from build123d import *

# Parameters (mm, degrees)
SKETCH1_W                 = 37.50000004
SKETCH1_H                 = 31.999999963
BOSS_EXTRUDE1_DEPTH       = 3
SKETCH2_W                 = 6
SKETCH2_H                 = 61.71460232
BOSS_EXTRUDE2_DEPTH       = 25.662738028
SKETCH3_W                 = 63.162738068
SKETCH3_H                 = 6
BOSS_EXTRUDE3_DEPTH       = 5.000000037
SKETCH4_W                 = 63.162738068
SKETCH4_H                 = 6
BOSS_EXTRUDE4_DEPTH       = 8
SKETCH5_W                 = 6
SKETCH5_H                 = 74.714602357
BOSS_EXTRUDE5_DEPTH       = 55.76390052
CUT_EXTRUDE1_DEPTH        = 2.499999998
SKETCH7_W                 = 6
SKETCH7_H                 = 32.514602357
CUT_EXTRUDE2_DEPTH        = 18.3
SKETCH8_W                 = 6
SKETCH8_H                 = 29.714602357
CUT_EXTRUDE3_DEPTH        = 2.5
SKETCH9_W                 = 6
SKETCH9_H                 = 46.714602358
CUT_EXTRUDE4_DEPTH        = 20.968950764
SKETCH10_W                = 6
SKETCH10_H                = 46.714602357
CUT_EXTRUDE5_DEPTH        = 32.770113219
SKETCH11_W                = 20.8
SKETCH11_H                = 19.200000012
BOSS_EXTRUDE6_DEPTH       = 4
SKETCH12_W                = 32.5
SKETCH12_H                = 22
CUT_EXTRUDE6_DEPTH        = 187.686043948
SKETCH13_W                = 13.3
SKETCH13_H                = 9.2
CUT_EXTRUDE7_DEPTH        = 187.686043948
DRAFT1_ANGLE              = -5
DRAFT2_ANGLE              = 5
F_4_CLEARANCE_HOLE1_D     = 3.4
F_4_CLEARANCE_HOLE1_DEPTH = 10
FILLET1_R                 = 1
FILLET2_R                 = 2.5
FILLET3_R                 = 5
CHAMFER1_SIZE             = 1


with BuildPart() as part:
    # Sketch1 → Boss-Extrude1 (new body)
    with BuildSketch(Plane.XY.offset(3)):
        with Locations((-62.281298008, 105.644197082)):
            Rectangle(SKETCH1_W, SKETCH1_H)
    extrude(amount=-BOSS_EXTRUDE1_DEPTH)

    # Sketch2 → Boss-Extrude2 (add)
    with BuildSketch(Plane(origin=(-43.531297988, 0, 0), x_dir=(0, 0, -1), z_dir=(1, 0, 0))):
        with Locations((0, 90.786895904)):
            Rectangle(SKETCH2_W, SKETCH2_H)
    extrude(amount=BOSS_EXTRUDE2_DEPTH)

    # Sketch3 → Boss-Extrude3 (add)
    with BuildSketch(Plane(origin=(0, 121.644197064, 0), x_dir=(-1, 0, 0), z_dir=(0, 1, 0))):
        with Locations((49.449928994, 0)):
            Rectangle(SKETCH3_W, SKETCH3_H)
    extrude(amount=BOSS_EXTRUDE3_DEPTH)

    # Sketch4 → Boss-Extrude4 (add)
    with BuildSketch(Plane.XZ.offset(-59.929594744)):
        with Locations((-49.449928994, 0)):
            Rectangle(SKETCH4_W, SKETCH4_H)
    extrude(amount=BOSS_EXTRUDE4_DEPTH)

    # Sketch5 → Boss-Extrude5 (add)
    with BuildSketch(Plane.ZY.offset(81.031298028)):
        with Locations((0, 89.286895923)):
            Rectangle(SKETCH5_W, SKETCH5_H)
    extrude(amount=BOSS_EXTRUDE5_DEPTH)

    # Sketch6 → Cut-Extrude1 (cut)
    with BuildSketch(Plane(origin=(-81.031298028, 0, 0), x_dir=(0, 0, -1), z_dir=(1, 0, 0))):
        Polygon((0, 89.644197101), (-3, 89.644197101), (-3, 59.929594744), (3, 59.929594744), (3, 92.444197101), (0, 92.444197101), align=None)
    extrude(amount=-CUT_EXTRUDE1_DEPTH, mode=Mode.SUBTRACT)

    # Sketch7 → Cut-Extrude2 (cut)
    with BuildSketch(Plane(origin=(-83.531298026, 0, 0), x_dir=(0, 0, -1), z_dir=(1, 0, 0))):
        with Locations((0, 76.186895922)):
            Rectangle(SKETCH7_W, SKETCH7_H)
    extrude(amount=-CUT_EXTRUDE2_DEPTH, mode=Mode.SUBTRACT)

    # Sketch8 → Cut-Extrude3 (cut)
    with BuildSketch(Plane.ZY.offset(43.531297988)):
        with Locations((0, 74.786895923)):
            Rectangle(SKETCH8_W, SKETCH8_H)
    extrude(amount=-CUT_EXTRUDE3_DEPTH, mode=Mode.SUBTRACT)

    # Sketch9 → Cut-Extrude4 (cut)
    with BuildSketch(Plane.ZY.offset(41.031297988)):
        with Locations((-1.31e-07, 83.286895949)):
            Rectangle(SKETCH9_W, SKETCH9_H)
    extrude(amount=-CUT_EXTRUDE4_DEPTH, mode=Mode.SUBTRACT)

    # Sketch10 → Cut-Extrude5 (cut)
    with BuildSketch(Plane(origin=(-101.831298026, 0, 0), x_dir=(0, 0, -1), z_dir=(1, 0, 0))):
        with Locations((0, 83.286895923)):
            Rectangle(SKETCH10_W, SKETCH10_H)
    extrude(amount=-CUT_EXTRUDE5_DEPTH, mode=Mode.SUBTRACT)

    # Sketch11 → Boss-Extrude6 (add)
    with BuildSketch(Plane(origin=(0, 0, -3), x_dir=(-1, 0, 0), z_dir=(0, 0, -1))):
        with Locations((91.431298026, 102.044197107)):
            Rectangle(SKETCH11_W, SKETCH11_H)
    extrude(amount=BOSS_EXTRUDE6_DEPTH)

    # Sketch12 → Cut-Extrude6 (cut, through all)
    with BuildSketch(Plane.XY.offset(3)):
        with Locations((-62.281298026, 105.644197101)):
            Rectangle(SKETCH12_W, SKETCH12_H)
    extrude(amount=-CUT_EXTRUDE6_DEPTH, mode=Mode.SUBTRACT)

    # Sketch13 → Cut-Extrude7 (cut, through all)
    with BuildSketch(Plane.XY.offset(3)):
        with Locations((-90.181298026, 102.044197101)):
            Rectangle(SKETCH13_W, SKETCH13_H)
    extrude(amount=-CUT_EXTRUDE7_DEPTH, mode=Mode.SUBTRACT)

    # Draft1
    draft1_faces = [part.faces().sort_by_distance(p)[0] for p in [
        (-20.062347224, 83.286895949, -1.31e-07),
        (-134.601411245, 83.286895923, 0),
    ]]
    draft(draft1_faces, Plane(origin=(0, 59.929594744, 0), x_dir=(1, 0, 0), z_dir=(0, 1, 0)), DRAFT1_ANGLE)

    # Draft2
    draft2_faces = [part.faces().sort_by_distance(p)[0] for p in [
        (-136.795198548, 89.286895923, 0),
        (-17.86855996, 89.286895923, 0),
    ]]
    draft(draft2_faces, Plane.ZX.offset(126.644197101), DRAFT2_ANGLE)

    # #4 Clearance Hole1
    with Locations(Plane.XY.offset(3)):
        with Locations((-21.533884656, 122.644197101), (-133.129873852, 122.644197101), (-138.966645249, 55.929594744), (-15.697113258, 55.929594744)):
            Hole(F_4_CLEARANCE_HOLE1_D / 2, depth=F_4_CLEARANCE_HOLE1_DEPTH)

    # Fillet1
    fillet1_edges = [part.edges().sort_by_distance(p)[0] for p in [
        (-83.531298026, 89.644197101, 1.5),
        (-101.831298026, 92.444197101, -2),
        (-83.531298026, 92.444197101, 1.5),
    ]]
    fillet(fillet1_edges, radius=FILLET1_R)

    # Fillet2
    fillet2_edges = [part.edges().sort_by_distance(p)[0] for p in [
        (-17.86855996, 126.644197101, 0),
        (-11.331879254, 51.929594744, 0),
        (-136.795198548, 126.644197101, 0),
        (-143.331879255, 51.929594744, 0),
    ]]
    fillet(fillet2_edges, radius=FILLET2_R)

    # Fillet3
    fillet3_edges = [part.edges().sort_by_distance(p)[0] for p in [
        (-101.831298026, 106.644197101, 0),
        (-41.031297988, 106.644197128, -1.31e-07),
        (-41.031297988, 89.644197101, 0),
        (-20.062347226, 59.92959477, 0),
        (-24.149345354, 106.644197128, 0),
        (-130.514413118, 106.644197101, 0),
        (-134.601411243, 59.92959477, 0),
    ]]
    fillet(fillet3_edges, radius=FILLET3_R)

    # Chamfer1
    chamfer1_edges = [part.edges().sort_by_distance(p)[0] for p in [
        (-46.031298026, 105.644197101, 3),
        (-62.281298026, 116.644197101, 3),
        (-78.531298026, 105.644197101, 3),
        (-62.281298026, 94.644197101, 3),
        (-90.181298026, 106.644197101, 3),
        (-96.831298026, 102.044197101, 3),
        (-90.181298026, 97.444197101, 3),
        (-83.531298026, 102.044197101, 3),
        (-13.997113258, 55.929594744, 3),
        (-137.266645249, 55.929594744, 3),
        (-131.429873852, 122.644197101, 3),
        (-19.833884656, 122.644197101, 3),
        (-92.681298026, 92.444197101, 3),
        (-83.531298026, 91.044197101, 3),
        (-64.281298007, 89.644197101, 3),
        (-101.538404807, 92.73709032, 3),
        (-83.238404807, 89.93709032, 3),
        (-83.824191245, 92.151303882, 3),
        (-77.331879254, 51.929594744, 3),
        (-77.331879254, 126.644197101, 3),
        (-140.044476053, 89.504785279, 3),
        (-14.619282455, 89.504785279, 3),
        (-136.193346132, 125.987390443, 3),
        (-18.470412376, 125.987390443, 3),
        (-142.446801344, 52.740619225, 3),
        (-12.216957164, 52.740619225, 3),
        (-116.382027637, 106.644197101, 3),
        (-101.831298026, 97.544197101, 3),
        (-32.381149606, 106.644197128, 2.999999869),
        (-41.031297988, 98.144197115, 2.999999869),
        (-22.143971987, 83.722674663, 3),
        (-61.031298008, 59.929594744, 3),
        (-132.519786483, 83.722674649, 3),
        (-42.495764082, 91.108663195, 3),
        (-103.29576412, 105.179731007, 3),
        (-39.566831894, 105.179731034, 3),
        (-21.832503047, 61.551643732, 3),
        (-25.353050186, 105.330583812, 3),
        (-129.310708286, 105.330583785, 3),
        (-132.831255421, 61.551643732, 3),
    ]]
    chamfer(chamfer1_edges, length=CHAMFER1_SIZE - 0.0001)  # a hair under: the kernel refuses the full size


solid = part.part
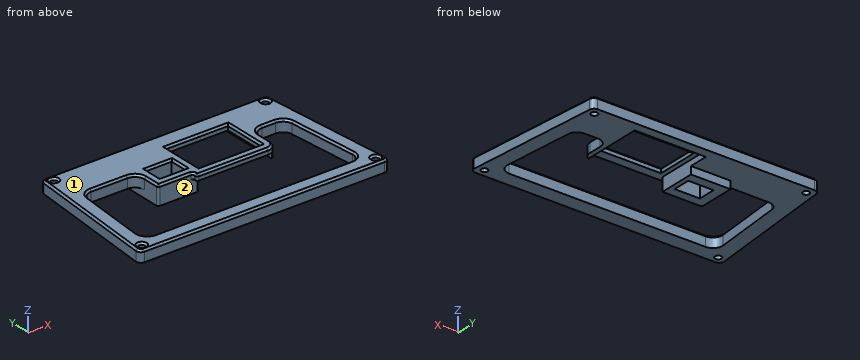
Read the model definition and answer for the solid it produces. Units are mm, in the model's axes. Face numbers are marked on the shaded views. Round coordinates to 2 decimals unless told otherwise and drop trailing zeros. Loops run counter-clockwise (first coordinate to the right, second up) from the corner with the lowest first, then second, coordinate; pieces in that order, holes last.
Q1. Determine the mould class of the marked faces 1 and 2 for opening direction Y: released by +Y, released by -Y, zero draft, split by the parting line, or undercut.
Q2. Consider probe 1 along Y at (x, z) = (-60.5, 1.5); probe 2 along Y at (x, z) = (-33.5, 0.5); probe 3 along Y at (x, z) = (-94, -4). Determine where each line is inside the solid, lowest interval first.
Q3. Section B-B on x = -122 is taken. Write down the section's boundary in (y, z), and give its area (3 significant figures).
Q4. Section C-C on y = 69 is taken. Write down the section's boundary in (x, z), and give its area (3 significant figures).
Q5. Section A-A on x = -52 is taken. Write down the section's boundary in (y, z).
Q6. Each of these flat-tipped pins is pushed along its axis until it touches: pin 1 (4.5 mm diameter, centred on x = -95, z = -5.5, fed in from +Y); pin 2 (5.5 mm diameter, centred on y = 113, z = -2.5, fed in from +X); pin 3 (1 mm diameter, centred on y = 102.5, z = 1.5, fed in from +X). Where does it stop, or does it pass through?
Output:
1. face 1: zero draft
1. face 2: undercut
2. probe 1: y = 51.93 to 59.93, 89.64 to 94.64, 116.64 to 126.64
2. probe 2: y = 51.93 to 59.93, 106.64 to 126.64
2. probe 3: y = 92.44 to 97.44, 106.64 to 111.64
3. outline: (51.93, -3) - (59.93, -3) - (59.93, 2) - (58.93, 3) - (52.93, 3) - (51.93, 2) - close; (106.64, -3) - (126.64, -3) - (126.64, 2) - (125.64, 3) - (107.64, 3) - (106.64, 2) - close
3. area: 166 mm2
4. outline: (-141.84, -3) - (-133.81, -3) - (-133.81, 2) - (-134.81, 3) - (-140.83, 3) - (-141.84, 2) - close; (-20.86, -3) - (-12.83, -3) - (-12.83, 2) - (-13.83, 3) - (-19.85, 3) - (-20.86, 2) - close
4. area: 94.4 mm2
5. outline: (51.93, -3) - (59.93, -3) - (59.93, 2) - (58.93, 3) - (52.93, 3) - (51.93, 2) - close; (89.64, 0) - (94.64, 0) - (94.64, 2) - (93.64, 3) - (90.64, 3) - (89.64, 2) - close; (116.64, 0) - (121.64, 0) - (121.64, -3) - (126.64, -3) - (126.64, 2) - (125.64, 3) - (117.64, 3) - (116.64, 2) - close
6. pin 1: stops at y = 111.64
6. pin 2: stops at x = -16.43
6. pin 3: stops at x = -15.71
